```python
from build123d import *

# Parameters (mm, degrees)
F3_W     = 14.659638
F3_H     = 4.675124
F4_DEPTH = 10


with BuildPart() as f2:
    # F0 (on Front) → F2 (revolve)
    with BuildSketch(Plane.XZ):
        Polygon((0, 12.7), (0, 0), (12.7, 0), align=None)
    revolve(axis=Axis((0, 0, 19.931149), (0, 0, 1)))

    # F3 (on Top) → F4 (join)
    with BuildSketch(Plane.XY):
        Rectangle(F3_W, F3_H)
    extrude(amount=-F4_DEPTH)


solid = f2.part
```
For this review, take the finished solid that the model builds, in its own axes (mm). A direction names the side the tool comes from. Round coordinates to 2 decimals unless told otherwise and drop trailing zeros. Write each loop counter-clockwise with the first axis right and the second up, starting at its lowest first coordinate (ties: lowest second). Pieces come first, ordered by that corner, then holes. Notation, with made-up numbers: (25.25, 21.5) - (45.25, 21.5) arc R15 ccw to (45.25, 46.5) - close; hole circle Ø2 at (56.25, 23). An arc over 180 degrees is marked (long way). Write each question's results on one line, items separated by ' | '.
Item 1: For pin 1 (1 mm diameter, centred on x = -8.5, y = 6, fed in from -Z); pin 2 (3 mm diameter, centred on x = 2.5, z = -3.5, fed in from -Y); pin 3 (3.5 mm diameter, centred on y = -0.5, z = -3.5, fed in from -X); pin 4 (1.5 mm diameter, centred on x = 9, z = -7, fed in from -Y), all flat-tipped, find the tip position at first contact; note any pin that passes through.
Calculated:
pin 1: stops at z = 0 | pin 2: stops at y = -2.34 | pin 3: stops at x = -7.33 | pin 4: passes through
Item 2: Take a section at A-A on z = 8.5. State the section outline as (x, y) points, then the cut area to 3 significant figures.
Calculated:
outline: circle Ø8.4 at (0, 0) | area: 55.4 mm^2
Item 3: Take a section at C-C on z = -2.5. State the section outline as (x, y) points, then the cut area to 3 significant figures.
Calculated:
outline: (-7.33, -2.34) - (7.33, -2.34) - (7.33, 2.34) - (-7.33, 2.34) - close | area: 68.5 mm^2
Item 4: Take a section at B-B on z = 3.5. State the section outline as (x, y) points, then the cut area to 3 significant figures.
Calculated:
outline: circle Ø18.4 at (0, 0) | area: 266 mm^2
Item 5: For faces 1 (the face through (0, -2.338, -5)), 2 (the face through (7.33, 0, -5)), 3 (the face through (-7.33, 0, -5)), list the 3-axis set-ups (+Z, -Z, +X, -X, +Y, -Y) from which the entire face can be reached by the end or side of a thin tool; tool diameter is ignored.
Calculated:
face 1: -Z, +X, -X, -Y | face 2: -Z, +X, +Y, -Y | face 3: -Z, -X, +Y, -Y
Item 6: To check wall thickness, follow line 1 along X through (y, z) = (-2.25, -4.25); line 2 along Y through (x, z) = (-2, -5); line 3 along X through (y, z) = (-2.5, 7.25). State the ranges of each line that lie inside material, in increasing order. Write a range as from..to.
Calculated:
line 1: x = -7.33..7.33 | line 2: y = -2.34..2.34 | line 3: x = -4.84..4.84
